Can you work these out from the model? Positions are in its coordinate system, mm. Face numbers are marked on the shaded views. Coordinates: 2 decimals unless noted, no trailing zeros. Order: outer loops, then holes, each group sorted by start corner. A loop starts at its lowest first (then second) coordinate and runs counter-clockwise, first axis right, second up. Notation, with made-up numbers: (47, 73) -> (67, 73) arc R20 cw to (67, 88) -> close; hole circle Ø8 at (28.25, 76.5). An arc over 180 degrees is marked (long way). Answer as a JSON object with one key per item and string values. Group by question number.
(1) For pin 1 (6 mm diameter, centred on x = -3, y = 11, fed in from -Z); pin 2 (4 mm diameter, centred on x = -14.5, y = 1.5, fed in from +Z); pin 3 (3 mm diameter, centred on x = -1.5, y = 2.5, fed in from -Z), each with a flat end and sliding along its axis, tell me the tip position at first contact or that it passes through.
(2) I want a section at B-B, the plane z = 8. List the corners of the cut face in (x, y) for me, plus the area to 3 significant figures.
(3) I want a section at A-A, the plane z = -15. List the corners of the cut face in (x, y) for me.
(4) I need wall thicknesses on line 1 (Y direction, x = -2.5, z = -3); line 2 (Z direction, x = 17, y = -14.5); line 3 (Z direction, x = 20, y = 3). Which ranges of each line are inside material? Lowest first, please.
(5) If we mould it in two halves opening along Z, with no side actions, what happens to the marked faces 1, 2 and 3? For each: pulls with the +Z half, pulls with the -Z half, needs draft (parallel to the pull), parting line crosses it, or undercut.
from build123d import *

# Parameters (mm, degrees)
F3_W      = 12.7
F3_H      = 12.7
F4_DEPTH  = 78.486
F6_DEPTH  = 56.134
F8_DEPTH  = 25.4
F10_DEPTH = 25.4


# Not quite as in the source:
# - a feature names something its author has since deleted; it is built from what else it names


with BuildPart() as f1:
    # F0 (on Right) → F1 (revolve)
    with BuildSketch(Plane.YZ):
        Polygon((0, 43.3274172246), (-29.0957745165, 0), (0, 0), align=None)
    revolve(axis=Axis((0, 0, 21.6637086123), (0, 0, -1)))

    # F3 (on face) → F4 (join)
    with BuildSketch(Plane(origin=(0, 0, 0), x_dir=(1, 0, 0), z_dir=(0, 0, -1))):
        with Locations((-0.3540940419, -0.2081472591)):
            Rectangle(F3_W, F3_H)
    extrude(amount=F4_DEPTH)

    # F5 (on face) → F6 (join)
    with BuildSketch(Plane.YZ.offset(5.9959059581)):
        Polygon((0, -7.9661617056), (0, -3.1097470783), (0, 0), (-6.1418527409, 0), (-6.1418527409, -78.486), (0, -78.486), (0, -77.0541617056), (0, -72.1977470783), (0, -59.7821617056), (0, -54.9257470783), (0, -42.5101617056), (0, -37.6537470783), (0, -25.2381617056), (0, -20.3817470783), align=None)
        Polygon((3.7682792172, -3.1097470783), (0, -3.1097470783), (0, -7.9661617056), (3.7682792172, -7.9661617056), (6.5581472591, -5.6115360931), align=None)
        Polygon((3.7682792172, -20.3817470783), (0, -20.3817470783), (0, -25.2381617056), (3.7682792172, -25.2381617056), (6.5581472591, -22.8835360931), align=None)
        Polygon((3.7682792172, -42.5101617056), (6.5581472591, -40.1555360931), (3.7682792172, -37.6537470783), (0, -37.6537470783), (0, -42.5101617056), align=None)
        Polygon((3.7682792172, -59.7821617056), (6.5581472591, -57.4275360931), (3.7682792172, -54.9257470783), (0, -54.9257470783), (0, -59.7821617056), align=None)
        Polygon((0, -72.1977470783), (0, -77.0541617056), (3.7682792172, -77.0541617056), (6.5581472591, -74.6995360931), (3.7682792172, -72.1977470783), align=None)
    extrude(amount=-F6_DEPTH)

    # F5 (on face) → F8 (cut)
    with BuildSketch(Plane.YZ.offset(5.9959059581)):
        Polygon((0, 0), (0, -3.1097470783), (3.7682792172, -3.1097470783), (6.5581472591, -5.6115360931), (6.5581472591, 0), align=None)
        Polygon((3.7682792172, -7.9661617056), (0, -7.9661617056), (0, -20.3817470783), (3.7682792172, -20.3817470783), (6.5581472591, -22.8835360931), (6.5581472591, -5.6115360931), align=None)
        Polygon((6.5581472591, -40.1555360931), (6.5581472591, -22.8835360931), (3.7682792172, -25.2381617056), (0, -25.2381617056), (0, -37.6537470783), (3.7682792172, -37.6537470783), align=None)
        Polygon((6.5581472591, -57.4275360931), (6.5581472591, -40.1555360931), (3.7682792172, -42.5101617056), (0, -42.5101617056), (0, -54.9257470783), (3.7682792172, -54.9257470783), align=None)
        Polygon((6.5581472591, -74.6995360931), (6.5581472591, -57.4275360931), (3.7682792172, -59.7821617056), (0, -59.7821617056), (0, -72.1977470783), (3.7682792172, -72.1977470783), align=None)
        Polygon((0, -77.0541617056), (0, -78.486), (6.5581472591, -78.486), (6.5581472591, -74.6995360931), (3.7682792172, -77.0541617056), align=None)
    extrude(amount=-F8_DEPTH, mode=Mode.SUBTRACT)

    # F9 (on face) → F10 (cut)
    with BuildSketch(Plane.XZ.offset(6.1418527409)):
        Polygon((-4.6626133844, -78.486), (-4.6626133844, 0), (-28.4401431013, 0), (-50.1380940419, 0), (-50.1380940419, -78.486), align=None)
    extrude(amount=-F10_DEPTH, mode=Mode.SUBTRACT)


with BuildPart() as f2:
    # F0 (on Right) → F2 (revolve)
    with BuildSketch(Plane.YZ):
        Polygon((122.2083866596, 0), (151.3041611761, 0), (122.2083866596, 43.3274172246), align=None)
    revolve(axis=Axis((0, 122.2083866596, 21.6637086123), (0, 0, -1)))


solid = f1.part
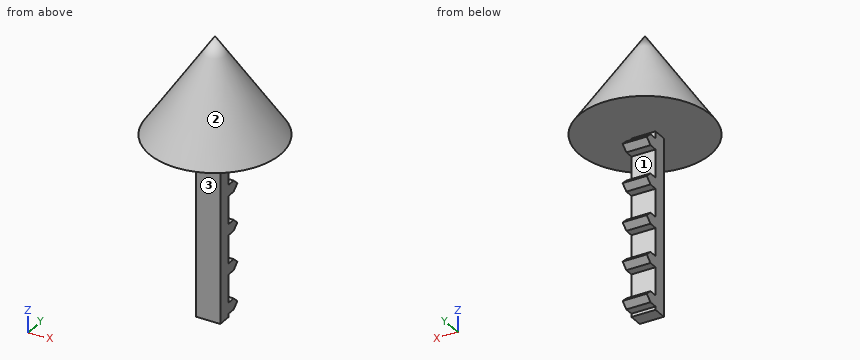
Computed values:
{
 "1": {"pin 1": "stops at z = 0", "pin 2": "stops at z = 24.6", "pin 3": "stops at z = -77.05"},
 "2": {"outline": "circle Ø47.45 at (0, 0)", "area": "1,770 mm2"},
 "3": {"outline": "(-4.66, -6.14) -> (6, -6.14) -> (6, 0) -> (-4.66, 0) -> close"},
 "4": {"line 1": "y = -6.14 to 0", "line 2": "z = 0 to 10.05", "line 3": "z = 0 to 13.21"},
 "5": {"face 1": "undercut", "face 2": "pulls with the +Z half", "face 3": "needs draft"}
}
